Verification items for the finished model (mm, model axes). A direction names the side the tool comes from. Coordinates: 2 decimals unless noted, no trailing zeros. Loops run counter-clockwise (first coordinate to the right, second up) from the corner with the lowest first, then second, coordinate; pieces in that order, holes last.
Q1. Mould release check, pull along Y, two halves, no side actions. Record for faces 1 (the face through (-113, 0, 2)), 2 (the face through (72, 36.504, 3)), 3 (the face through (31.504, -41.578, 2.535)): +Y half, -Y half, draft (parallel to the pull), parting line (faces both ways), or undercut.
Q2. Go/stop test with flat-tipped pins: P1, Ø4, axis at x = -42, y = 25.5, coming from the -Z side; P2, Ø1.8, axis at x = 42, y = 25.5, coming from the -Z side. Record where each tip stops, or that it passes through.
Q3. Access from +Z, -Z, +X, -X, +Y, -Y to the whole of each face (thin tool, end or side, straight path). Record for faces 4 (the face through (72, -36.504, 3)), 5 (the face through (-23.504, 41.578, 2.535)), 6 (the face through (0, -30.004, 3)).
Q4. Sectioned sample at A-A (x = -82). Enter the section's corners in (y, z).
Q5. Material ranges on probe 1 along Y at (x, z) = (42, 3.6); probe 2 along Y at (x, z) = (-86, 1.45); probe 3 along X at (y, z) = (34, 1.25), recorded low to high.
```python
from build123d import *

# Parameters (mm, degrees)
PAD_DEPTH       = 5
SKETCH001_R     = 3
SKETCH001_R_2   = 1.7
SKETCH001_R_3   = 1.5
SKETCH001_W     = 60
SKETCH001_H     = 20
POCKET_DEPTH    = 5.001
FILLET_R        = 5
FILLET001_R     = 20
SKETCH002_R     = 3.5
POCKET001_DEPTH = 2


with BuildPart() as part:
    # Sketch → Pad (new body)
    with BuildSketch(Plane.XY):
        with BuildLine():
            ThreePointArc((-22, -30.983867), (0, -38), (22, -30.983867))
            Line((22, -43.003867), (22, -30.983867))
            Line((113, -43.003867), (22, -43.003867))
            Line((113, 43.003867), (113, -43.003867))
            Line((22, 43.003867), (113, 43.003867))
            Line((22, 30.983867), (22, 43.003867))
            ThreePointArc((22, 30.983867), (0, 38), (-22, 30.983867))
            Line((-22, 43.003867), (-22, 30.983867))
            Line((-113, 43.003867), (-22, 43.003867))
            Line((-113, -43.003867), (-113, 43.003867))
            Line((-22, -43.003867), (-113, -43.003867))
            Line((-22, -30.983867), (-22, -43.003867))
        make_face()
    extrude(amount=PAD_DEPTH)

    # Sketch001 (on Face14 of Pad) → Pocket (cut, through all)
    with BuildSketch(Plane.XY.offset(5)):
        with Locations((0, -17)):
            Circle(SKETCH001_R)
        with Locations((0, 7)):
            Circle(SKETCH001_R_2)
        with Locations((42, 25.496133)):
            Circle(SKETCH001_R_3)
        with Locations((42, -36.003867)):
            Circle(SKETCH001_R_3)
        with Locations((-42, 25.496133)):
            Circle(SKETCH001_R_3)
        with Locations((-42, -36.003867)):
            Circle(SKETCH001_R_3)
        with Locations((0, -40.003867)):
            Rectangle(SKETCH001_W, SKETCH001_H)
        with BuildLine():
            ThreePointArc((-92, 39.503867), (-93.5, 38.003867), (-92, 36.503867))
            Line((-92, 36.503867), (-52, 36.503867))
            ThreePointArc((-52, 36.503867), (-50.5, 38.003867), (-52, 39.503867))
            Line((-52, 39.503867), (-92, 39.503867))
        make_face()
        with BuildLine():
            ThreePointArc((52, 39.503867), (50.5, 38.003867), (52, 36.503867))
            Line((52, 36.503867), (92, 36.503867))
            ThreePointArc((92, 36.503867), (93.5, 38.003867), (92, 39.503867))
            Line((92, 39.503867), (52, 39.503867))
        make_face()
        with BuildLine():
            ThreePointArc((-92, -36.503867), (-93.5, -38.003867), (-92, -39.503867))
            Line((-92, -39.503867), (-52, -39.503867))
            ThreePointArc((-52, -39.503867), (-50.5, -38.003867), (-52, -36.503867))
            Line((-52, -36.503867), (-92, -36.503867))
        make_face()
        with BuildLine():
            ThreePointArc((52, -36.503867), (50.5, -38.003867), (52, -39.503867))
            Line((52, -39.503867), (92, -39.503867))
            ThreePointArc((92, -39.503867), (93.5, -38.003867), (92, -36.503867))
            Line((92, -36.503867), (52, -36.503867))
        make_face()
    extrude(amount=-POCKET_DEPTH, mode=Mode.SUBTRACT)

    # Fillet
    fillet_edges = [part.edges().sort_by_distance(p)[0] for p in [
        (22, 43.003867, 2.5),
        (-22, 43.003867, 2.5),
        (30, -43.003867, 2.5),
        (-30, -43.003867, 2.5),
    ]]
    fillet(fillet_edges, radius=FILLET_R)

    # Fillet001
    fillet001_edges = [part.edges().sort_by_distance(p)[0] for p in [
        (-113, 43.003867, 2.5),
        (-113, -43.003867, 2.5),
        (113, 43.003867, 2.5),
        (113, -43.003867, 2.5),
    ]]
    fillet(fillet001_edges, radius=FILLET001_R)

    # Sketch002 (on Face1 of Fillet001) → Pocket001 (cut)
    with BuildSketch(Plane(origin=(0, 0, 0), x_dir=(1, 0, 0), z_dir=(0, 0, -1))):
        with Locations((-42, -25.496133)):
            Circle(SKETCH002_R)
        with Locations((-42, 36.003867)):
            Circle(SKETCH002_R)
        with Locations((42, 36.003867)):
            Circle(SKETCH002_R)
        with Locations((42, -25.496133)):
            Circle(SKETCH002_R)
    extrude(amount=-POCKET001_DEPTH, mode=Mode.SUBTRACT)


solid = part.part
```
Geometry check:
1. face 1: draft
1. face 2: undercut
1. face 3: -Y half
2. P1: stops at z = 2
2. P2: passes through
3. face 4: +Z, -Z
3. face 5: +Z, -Z, +Y
3. face 6: +Z, -Z, -Y
4. outline: (-43, 0) - (-39.5, 0) - (-39.5, 5) - (-43, 5) - close; (-36.5, 0) - (36.5, 0) - (36.5, 5) - (-36.5, 5) - close; (39.5, 0) - (43, 0) - (43, 5) - (39.5, 5) - close
5. probe 1: y = -43 to -37.5, -34.5 to 24, 27 to 43
5. probe 2: y = -43 to -39.5, -36.5 to 36.5, 39.5 to 43
5. probe 3: x = -109.71 to -22, -16.97 to 16.97, 22 to 109.71
